Autodesk Inventor part; units mm, degrees
ref_plane "YZ Plane" through (0, 0, 0) normal (1, 0, 0) x (0, 1, 0)
ref_plane "XZ Plane" through (0, 0, 0) normal (0, 1, 0) x (-1, 0, 0)
ref_plane "XY Plane" through (0, 0, 0) normal (0, 0, 1) x (1, 0, 0)
sketch "Sketch1" plane through (0, 0, 0) normal (0, 1, 0) x (-1, 0, 0)
  circle A0 centre (0, 0) radius 11.5
  circle A1 centre (0, 0) radius 15.125
  line L0 (0, 15.125) -> (15.125, 15.125)
  line L1 (0, -15.125) -> (15.125, -15.125)
  line L2 (15.125, 0) -> (15.125, 15.125)
  line L3 (15.125, 0) -> (15.125, -15.125)
  dimension "d0" = 23
  dimension "d1" = 30.25
extrude "Extrusion1" add sketch "Sketch1" along normal blind 36
sketch "Sketch2" plane through (-15.125, 0, -15.125) normal (-1, 0, 0) x (0, 0, 1)
  line L0 (0.2295, 33) -> (30.25, 33)
  line L1 (30.25, 0) -> (30.25, 36)
  line L2 (30.25, 3) -> (0, 3)
  line L3 (0, 0) -> (0, 36)
  line L4 (0, 0) -> (30.25, 0)
  line L5 (0, 36) -> (30.25, 36)
  line L6 (27.25, 36) -> (27.25, 0)
  line L7 (0, 33) -> (0.2295, 33)
  point P0 (15.125, 0)
  point P1 (15.125, 3)
  point P2 (15.125, 0)
  point P3 (15.125, 36)
  point P4 (15.2397, 33)
  point P5 (27.25, 33)
  point P6 (27.25, 3)
  dimension "d4" = 3
  dimension "d5" = 3
  dimension "d6" = 3
extrude "Extrusion2" add sketch "Sketch2" along normal blind 16.5 contours L7 L3 L5 L6 L0 | L6 L5 L1 L0 | L0 L1 L2 L6 | L6 L4 L3 L2 | L2 L1 L4 L6
sketch "Sketch3" plane through (-31.625, 0, -15.125) normal (-1, 0, 0) x (0, 0, 1)
  line L0 (30.25, 0) -> (30.25, 36)
  line L1 (0, 36) -> (30.25, 36)
  line L2 (30.25, 36) -> (30.25, 0)
  line L3 (30.25, 0) -> (0, 0)
  line L4 (0, 0) -> (0, 36)
  point P0 (15.125, 0)
extrude "Extrusion3" add sketch "Sketch3" along normal blind 3
sketch "Sketch4" plane through (-15.125, 3, 12.125) normal (0, 0, -1) x (-1, 0, 0)
  line L0 (16.5, 30) -> (16.5, 0)
  line L1 (0, 30) -> (16.5, 30)
  line L2 (16.5, 30) -> (16.5, 0)
  line L3 (16.5, 0) -> (0, 0)
  line L4 (0, 0) -> (0, 30)
  line L5 (0, 30) -> (16.5, 0)
  line L6 (0, 0) -> (16.5, 30)
  circle A0 centre (8.25, 15) radius 6.5
  point P0 (-15.125, -3)
  dimension "d11" = 13
extrude "Extrusion4" cut sketch "Sketch4" against normal blind 3 contours A0 L5 L6 | L6 L5 A0 | A0 L6 L5 | L5 L6 A0
properties part number "schimbator_support"
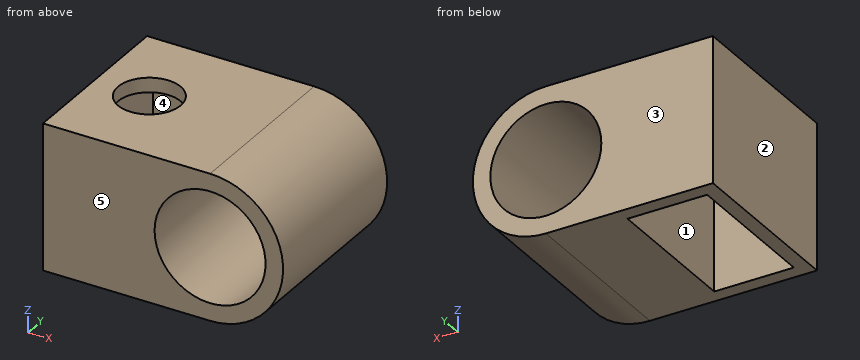
Verification items for the finished model (mm, model axes). Face numbers are marked on the shaded views. A direction names the side the tool comes from. Give positions to 0.01 mm unless a question says otherwise; leave off trailing zeros. Order: outer loops, then holes, each group sorted by start corner. A loop starts at its lowest first (then second) coordinate and runs counter-clockwise, first axis right, second up. Notation, with made-up numbers: (-29.75, -17) -> (23.25, -17) arc R24 cw to (23.25, 16) -> close; hole circle Ø10 at (-12.5, -33.75). An arc over 180 degrees is marked (long way). One line per item, written item: value.
(1) Sectioned sample at D-D on y = 29. Record the cut outline in (x, z) (3 decimals), then the cut area to 3 significant figures.
Final values:
outline: (-34.625, -15.125) -> (-31.625, -15.125) -> (-31.625, 12.125) -> (-15.125, 12.125) -> (-15.125, -15.125) -> (0, -15.125) arc R15.125 ccw to (0, 15.125) -> (-34.625, 15.125) -> close; hole circle Ø23 at (0, 0)
area: 542 mm^2
(2) Tool access check on the marked faces 4 and 5. Record the directions out of +Z, -Z, +X, -X, +Y, -Y that give a thin tool (end or side, any length) a straight path to the whole face; none if there is none.
Final values:
face 4: -Z
face 5: +Z, -Z, +X, -X, -Y
(3) Sectioned sample at C-C on x = -3.5. Record the cut outline in (y, z) (3 decimals), then the cut area to 3 significant figures.
Final values:
outline: (0, -15.125) -> (36, -15.125) -> (36, -10.954) -> (0, -10.954) -> close; (0, 10.954) -> (36, 10.954) -> (36, 15.125) -> (0, 15.125) -> close
area: 300 mm^2
(4) Sectioned sample at B-B on y = 18. Record the cut outline in (x, z) (3 decimals).
Final values:
outline: (-34.625, -15.125) -> (-31.625, -15.125) -> (-31.625, 12.125) -> (-29.875, 12.125) -> (-29.875, 15.125) -> (-34.625, 15.125) -> close; (-16.875, 12.125) -> (-15.125, 12.125) -> (-15.125, -15.125) -> (0, -15.125) arc R15.125 ccw to (0, 15.125) -> (-16.875, 15.125) -> close; hole circle Ø23 at (0, 0)
(5) Draft check along Y on the marked faces 1, 2 and 3. Enter one of: pulls with the +Y half, pulls with the -Y half, needs draft (parallel to the pull), parting line crosses it, or undercut.
Final values:
face 1: undercut
face 2: needs draft
face 3: pulls with the +Y half
(6) Sectioned sample at A-A on z = 0. Record the cut outline in (x, y) (3 decimals).
Final values:
outline: (-34.625, 0) -> (-11.5, 0) -> (-11.5, 36) -> (-34.625, 36) -> close; (11.5, 0) -> (15.125, 0) -> (15.125, 36) -> (11.5, 36) -> close; hole (-31.625, 3) -> (-15.125, 3) -> (-15.125, 33) -> (-31.625, 33) -> close
(7) Gauge pin test, flat ends, axial feed: pin 1 (5 mm diameter, centred on x = -24.5, y = 15.5, fed in from -Z); pin 2 (12 mm diameter, centred on y = 24.5, z = -11.5, fed in from +X); pin 3 (5 mm diameter, centred on y = 12.5, z = 7.5, fed in from +X). Record the tip position at first contact, or that the pin passes through.
Final values:
pin 1: through
pin 2: x = 14.09
pin 3: x = 14.27
(8) Scan lines: line 1 along Y through (x, z) = (-24.5, -13.5); line 2 along X through (y, z) = (32, -1.5) (3 decimals); line 3 along X through (y, z) = (20.5, -5.5) (1 decimal). Record each from-to range of solid material in increasing order. Write a range as [from, to].
Final values:
line 1: [0, 3], [33, 36]
line 2: [-34.625, -31.625], [-15.125, -11.402], [11.402, 15.05]
line 3: [-34.6, -31.6], [-15.1, -10.1], [10.1, 14.1]
